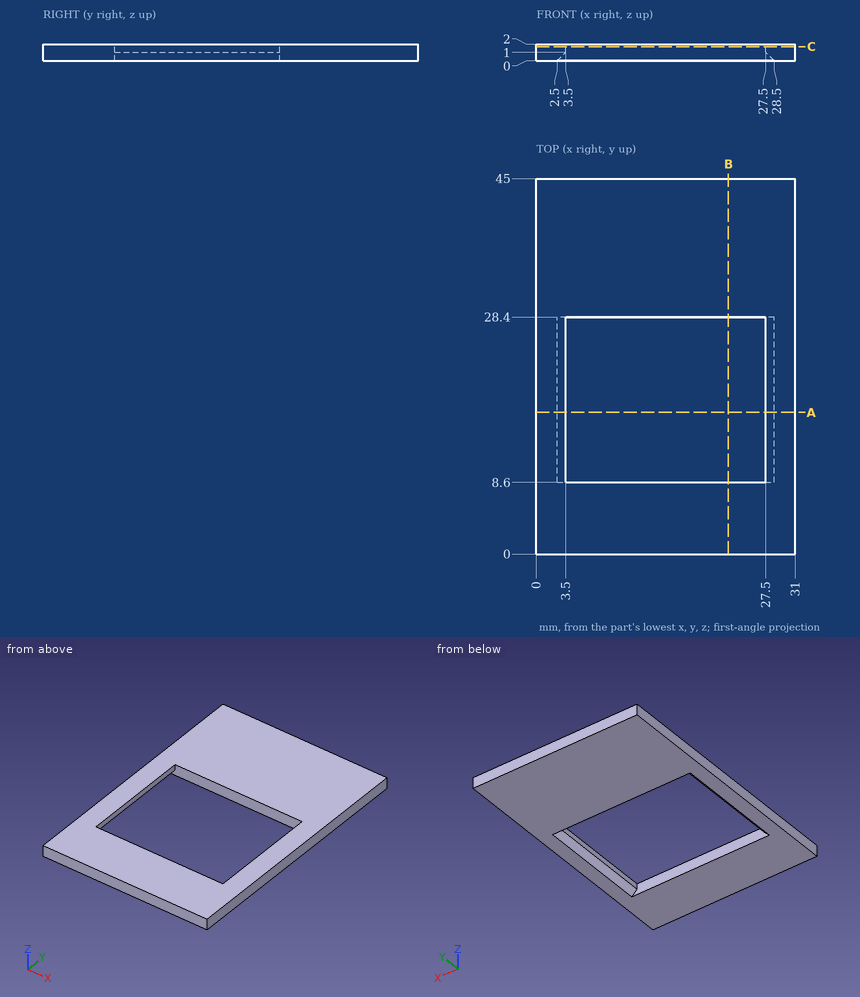
Here's the drawing with two shaded views (mm, measured from the low corner). I have some questions. Coordinates: 2 decimals unless noted, no trailing zeros. Loops run counter-clockwise (first coordinate to the right, second up) from the corner with the lowest first, then second, coordinate; pieces in that order, holes last. Notation, with made-up numbers: (19, 6.5) -> (34, 6.5) arc R20 cw to (34, 27.5) -> close; hole circle Ø5 at (-2.5, 71). An arc over 180 degrees is marked (long way). Put each result on its own line as item: value. Start each with the question number.
Q1. If I drill on line 1 (Y direction, x = 24.5, z = 0.45); line 2 (X direction, y = 27, z = 1.5); line 3 (X direction, y = 21, z = 0.1), over which ranges is the centre line in solid material (lowest first)? Write a range as [from, to].
Q2. I want a section at C-C (z = 1.7). Write out the boundary of the cut face in (x, y).
Q3. I want a section at B-B (x = 23). Write out the boundary of the cut face in (y, z).
Q4. I want a section at A-A (y = 17). Write out the boundary of the cut face in (x, z).
Taken from the geometry:
1. line 1: y = [0, 8.6], [28.4, 45]
1. line 2: x = [0, 3.5], [27.5, 31]
1. line 3: x = [0, 2.6], [28.4, 31]
2. outline: (0, 0) -> (31, 0) -> (31, 45) -> (0, 45) -> close; hole (3.5, 8.6) -> (27.5, 8.6) -> (27.5, 28.4) -> (3.5, 28.4) -> close
3. outline: (0, 0) -> (8.6, 0) -> (8.6, 2) -> (0, 2) -> close; (28.4, 0) -> (45, 0) -> (45, 2) -> (28.4, 2) -> close
4. outline: (0, 0) -> (2.5, 0) -> (3.5, 1) -> (3.5, 2) -> (0, 2) -> close; (27.5, 1) -> (28.5, 0) -> (31, 0) -> (31, 2) -> (27.5, 2) -> close
